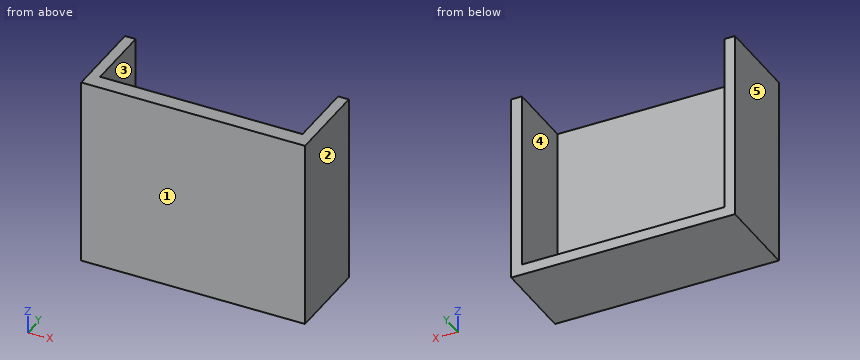
from build123d import *

# Parameters (mm, degrees)
SKETCH1_W           = 113.01
SKETCH1_H           = 95.57
BOSS_EXTRUDE1_DEPTH = 42.75
SKETCH3_W           = 102.21
SKETCH3_H           = 90.17
CUT_EXTRUDE1_DEPTH  = 34.75
SKETCH6_W           = 102.21
SKETCH6_H           = 8.948308689
CUT_EXTRUDE2_DEPTH  = 34.75


with BuildPart() as part:
    # Sketch1 → Boss-Extrude1 (new body)
    with BuildSketch(Plane(origin=(0, 0, 0), x_dir=(1, 0, 0), z_dir=(0, 1, 0))):
        Rectangle(SKETCH1_W, SKETCH1_H)
    extrude(amount=BOSS_EXTRUDE1_DEPTH)

    # Sketch3 → Cut-Extrude1 (cut)
    with BuildSketch(Plane(origin=(0, 42.75, 0), x_dir=(1, 0, 0), z_dir=(0, 1, 0))):
        with Locations((0, -2.692303692)):
            Rectangle(SKETCH3_W, SKETCH3_H)
    extrude(amount=-CUT_EXTRUDE1_DEPTH, mode=Mode.SUBTRACT)

    # Sketch6 → Cut-Extrude2 (cut)
    with BuildSketch(Plane(origin=(0, 42.75, 0), x_dir=(1, 0, 0), z_dir=(0, 1, 0))):
        with Locations((0, -47.777303693)):
            Rectangle(SKETCH6_W, SKETCH6_H)
    extrude(amount=-CUT_EXTRUDE2_DEPTH, mode=Mode.SUBTRACT)


solid = part.part
CAD build for the part. Positions are in the model's coordinates, mm. Face numbers are marked on the shaded views. A direction names the side the tool comes from. Coordinates: 2 decimals unless noted, no trailing zeros. Order: outer loops, then holes, each group sorted by start corner. A loop starts at its lowest first (then second) coordinate and runs counter-clockwise, first axis right, second up. Notation, with made-up numbers: (-35.5, 8) -> (20.5, 8) arc R21 ccw to (20.5, 38) -> close; hole circle Ø8 at (72.5, 6.25). An arc over 180 degrees is marked (long way). Answer in a Markdown table with one row per item.
1) Band-saw the part on C-C (x = -48.5). List the corners of the cut face in (y, z) (3 decimals).
Check values:
| item | result |
|---|---|
| outline | (0, -47.785) -> (42.75, -47.785) -> (42.75, -42.393) -> (8, -42.393) -> (8, 47.785) -> (0, 47.785) -> close |
2) Flat gauge pin, fed straight in: P1, Ø5, axis at x = -12.5, y = 35, coming from the +Z side. Where does the tip first touch, or does it go through?
Check values:
| item | result |
|---|---|
| P1 | z = -42.39 |
3) Which spindle directions (+Z, -Z, +X, -X, +Y, -Y) get a long thin tool onto all of the face, cutting with end or side? Do the marked faces 4 and 5. Say none if no direction does.
Check values:
| item | result |
|---|---|
| face 4 | +Z, +Y |
| face 5 | +Z, -Z, -X, +Y, -Y |
4) Band-saw the part on B-B (y = 25.5). List the corners of the cut face in (x, z) (3 decimals).
Check values:
| item | result |
|---|---|
| outline | (-56.505, -47.785) -> (56.505, -47.785) -> (56.505, 47.785) -> (51.105, 47.785) -> (51.105, -42.393) -> (-51.105, -42.393) -> (-51.105, 47.785) -> (-56.505, 47.785) -> close |
5) Band-saw the part on A-A (z = -5.5). List the corners of the cut face in (x, y) (3 decimals).
Check values:
| item | result |
|---|---|
| outline | (-56.505, 0) -> (56.505, 0) -> (56.505, 42.75) -> (51.105, 42.75) -> (51.105, 8) -> (-51.105, 8) -> (-51.105, 42.75) -> (-56.505, 42.75) -> close |
6) Drill centre lines: line 1 (X direction, y = 37.5, z = 7.5) (3 decimals); line 2 (Y direction, x = -35.5, z = 29.5); line 3 (Z direction, x = -23, y = 35.5) (3 decimals). Where is each one in solid material? Low to high.
Check values:
| item | result |
|---|---|
| line 1 | -56.505 to -51.105, 51.105 to 56.505 |
| line 2 | 0 to 8 |
| line 3 | -47.785 to -42.393 |
7) Mould opens along X. For the marked faces 1, 2 and 3 say: pulls with the +X half, pulls with the -X half, needs draft (parallel to the pull), parting line crosses it, or undercut.
Check values:
| item | result |
|---|---|
| face 1 | needs draft |
| face 2 | pulls with the +X half |
| face 3 | undercut |
